Input: dimensioned drawing with shaded views. Units: mm. Origin: part minimum x, y, z. A direction names the side the tool comes from. Round coordinates to 2 decimals unless told otherwise and drop trailing zeros. Loops run counter-clockwise (first coordinate to the right, second up) from the corner with the lowest first, then second, coordinate; pieces in that order, holes last. Notation, with made-up numbers: (-17.75, 8.5) - (32.25, 8.5) arc R9 cw to (32.25, 25.5) - close; hole circle Ø6 at (49, 17.25). An arc over 180 degrees is marked (long way). One line per question, with ' | ' between items. Start each with the question number.
1. Cut plane D-D (y = 42). Return loops of the section in (x, z).
2. Cut plane B-B (z = 40). Return loops of the section in (x, y) (1 decimal).
3. Pin query (flat end, axial travel): pin 1 (3 mm diameter, centred on x = 35, z = 9.5, fed in from +Y) (1 decimal); pin 2 (12 mm diameter, centred on x = 30.5, y = 26, fed in from +Z); pin 3 (1.5 mm diameter, centred on x = 35.5, y = 36, fed in from -Z). Return the tip coordinate at first contact, or that it passes through.
4. Cut plane A-A (y = 33). Return loops of the section in (x, z).
5. Access query for the marked faces 1, 2, 3, 4 and 5. Directions: +Z, -Z, +X, -X, +Y, -Y. A direction counts if a zero-diameter tool reaches every point of the face in a straight line with its end or side. Return the directions, or none.
6. Ray query, line 1 (Z direction, x = 7, y = 26.5); line 2 (Z direction, x = 23.5, y = 36.5). Return the intervals inside material, ascending.
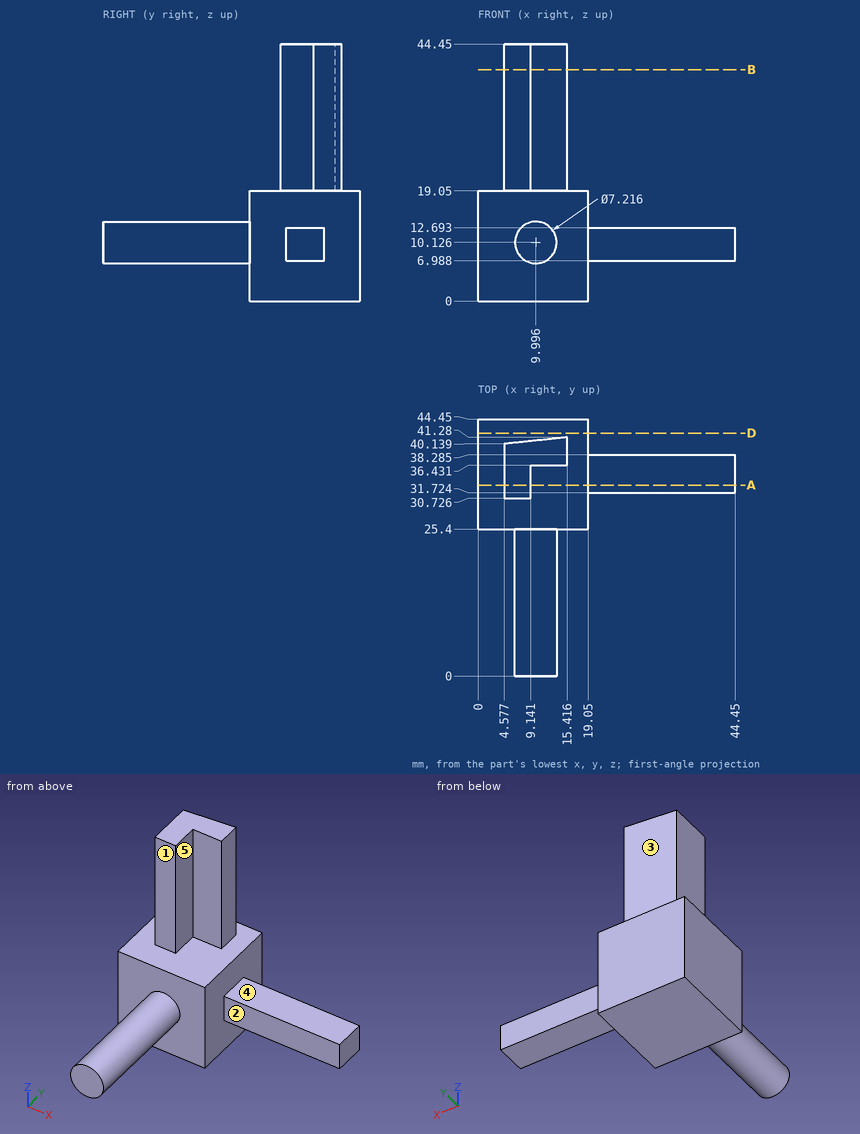
Answers follow:
1) outline: (0, 0) - (19.05, 0) - (19.05, 19.05) - (0, 19.05) - close
2) outline: (4.6, 30.7) - (9.1, 30.7) - (9.1, 36.4) - (15.4, 36.4) - (15.4, 41.3) - (4.6, 40.1) - close
3) pin 1: stops at y = 38.3 | pin 2: stops at z = 12.69 | pin 3: stops at z = 6.99
4) outline: (0, 0) - (19.05, 0) - (19.05, 6.99) - (44.45, 6.99) - (44.45, 12.69) - (19.05, 12.69) - (19.05, 19.05) - (9.14, 19.05) - (9.14, 44.45) - (4.58, 44.45) - (4.58, 19.05) - (0, 19.05) - close
5) face 1: +Z, +X, -X, -Y | face 2: +Z, -Z, +X, -Y | face 3: +Z, -X, +Y | face 4: +Z, +X, +Y, -Y | face 5: +Z, +X, -Y
6) line 1: z = 0 to 19.05 | line 2: z = 6.99 to 12.69
